Check sheet for the modelled part. Datum: model origin and axes. Units: mm. A direction names the side the tool comes from. Give positions to 0.01 mm unless a question says otherwise; leave off trailing zeros. Loops run counter-clockwise (first coordinate to the right, second up) from the corner with the lowest first, then second, coordinate; pieces in that order, holes last. Notation, with made-up numbers: (55.25, -5.5) - (60.25, -5.5) arc R16 cw to (60.25, 24.5) - close; hole circle Ø7 at (19.5, 43). An arc over 180 degrees is marked (long way). Use one line per item in the form item = value.
from build123d import *

# Parameters (mm, degrees)
CROQUIS1_R              = 1.5
SALIENTE_EXTRUIR1_DEPTH = 25
CROQUIS2_R              = 0.5
SALIENTE_EXTRUIR2_DEPTH = 1
CROQUIS3_R              = 0.5
SALIENTE_EXTRUIR3_DEPTH = 1


with BuildPart() as part:
    # Croquis1 → Saliente-Extruir1 (new body)
    with BuildSketch(Plane(origin=(0, 0, 0), x_dir=(0, 0, -1), z_dir=(1, 0, 0))):
        Circle(CROQUIS1_R)
    extrude(amount=SALIENTE_EXTRUIR1_DEPTH)

    # Croquis2 → Saliente-Extruir2 (add)
    with BuildSketch(Plane(origin=(25, 0, 0), x_dir=(0, 0, -1), z_dir=(1, 0, 0))):
        Circle(CROQUIS2_R)
    extrude(amount=SALIENTE_EXTRUIR2_DEPTH)

    # Croquis3 → Saliente-Extruir3 (add)
    with BuildSketch(Plane.ZY):
        Circle(CROQUIS3_R)
    extrude(amount=SALIENTE_EXTRUIR3_DEPTH)


solid = part.part
Item 1: Gauge pin test, flat end, axial feed: P1, Ø1, axis at x = 2, y = -1, coming from the -Z side. Record the tip position at first contact, or that the pin passes through.
Answer block:
P1 = -1.41
Item 2: Thickness scan on L1, parallel to X at y = -1.05, z = -0.7; L2, parallel to Z at x = 6.25, y = -0.1; L3, parallel to Y at x = 14.25, z = -1.05. Record the ranges inside material, lowest first.
Answer block:
L1 = 0 to 25
L2 = -1.5 to 1.5
L3 = -1.07 to 1.07
Item 3: Section check A-A on y = 0. Record the boundary of the cut face in (x, z), then the cut area to 3 significant figures.
Answer block:
outline = (-1, -0.5) - (0, -0.5) - (0, -1.5) - (25, -1.5) - (25, -0.5) - (26, -0.5) - (26, 0.5) - (25, 0.5) - (25, 1.5) - (0, 1.5) - (0, 0.5) - (-1, 0.5) - close
area = 77.0 mm2
Item 4: Section check D-D on z = -1.2. Record the boundary of the cut face in (x, y), then the cut area to 3 significant figures.
Answer block:
outline = (0, -0.9) - (25, -0.9) - (25, 0.9) - (0, 0.9) - close
area = 45.0 mm2
Item 5: Access from +Z, -Z, +X, -X, +Y, -Y to the whole of each face (thin tool, end or side, straight path). Record for faces 1 (the face through (25.493, -0.488, 0.108)), 2 (the face through (-1, 0, 0)), 3 (the face through (-0.493, -0.488, -0.108)).
Answer block:
face_1 = +X
face_2 = +Z, -Z, -X, +Y, -Y
face_3 = -X
Item 6: Section check C-C on x = 11. Record the boundary of the cut face in (y, z).
Answer block:
outline = circle Ø3 at (0, 0)
